Autodesk Inventor part; units mm, degrees
ref_plane "YZ Plane" through (0, 0, 0) normal (1, 0, 0) x (0, 1, 0)
ref_plane "XZ Plane" through (0, 0, 0) normal (0, 1, 0) x (-1, 0, 0)
ref_plane "XY Plane" through (0, 0, 0) normal (0, 0, 1) x (1, 0, 0)
sketch "Sketch1" plane through (0, 0, 0) normal (0, 0, 1) x (1, 0, 0)
  line L0 (0, 0) -> (25.4, 0)
  line L1 (25.4, 0) -> (25.4, 3.175)
  line L2 (3.175, 25.4) -> (0, 25.4)
  line L3 (0, 25.4) -> (0, 0)
  line L4 (3.175, 25.4) -> (3.175, 3.175)
  line L5 (3.175, 3.175) -> (25.4, 3.175)
  dimension "d1" = 25.4
  dimension "d2" = 3.175
  dimension "d3" = 3.175
  dimension "d4" = 25.4
extrude "Extrusion1" add sketch "Sketch1" along normal blind 139.7
fillet "Fillet1" radius 1.27 1 edges at (3.175, 25.4, 69.85)
fillet "Fillet2" radius 1.27 5 edges at (0, 25.4, 69.85) (25.4, 3.175, 69.85) (25.4, 0, 69.85) (0, 0, 69.85) (3.175, 3.175, 69.85)
sketch "Sketch2" plane through (4.445, 3.175, 0) normal (0, 1, 0) x (1, 0, 0)
  line L0 (0, -139.7) -> (19.685, -139.7)
  line L1 (19.685, 0) -> (0, 0)
  circle A0 centre (9.8425, -12.7) radius 3.175
  circle A1 centre (9.8425, -127) radius 3.175
  point P0 (-4.445, 0)
  dimension "d9" = 6.35
  dimension "d10" = 6.35
  dimension "d11" = 12.7
  dimension "d12" = 12.7
extrude "Extrusion2" cut sketch "Sketch2" against normal blind 152.4
sketch "Sketch3" plane through (3.175, 24.13, 139.7) normal (1, 0, 0) x (0, 0, -1)
  line L0 (44.45, -4.3683) -> (95.25, -4.3683)
  line L1 (95.25, -10.7183) -> (44.45, -10.7183)
  arc A0 (44.45, -4.3683) -> (44.45, -10.7183) centre (44.45, -7.5433) ccw
  arc A1 (95.25, -10.7183) -> (95.25, -4.3683) centre (95.25, -7.5433) ccw
  line L2 (139.7, -19.685) -> (139.7, 0)
  point P0 (139.7, -24.13)
  point P1 (0, 0)
  dimension "d20" = 44.45
  dimension "d21" = 50.8
  dimension "d22" = 139.7
extrude "Extrusion3" cut sketch "Sketch3" against normal blind 152.4
equation "\"d3\" = d2"
equation "\"d12\" = d11"
equation "\"d20\" = -0.5 * d21 + 0.5 * d22"
properties part number "BatteryMountSide"
Can you work these out from the model? Positions are in its coordinate system, mm. A direction names the side the tool comes from. Round coordinates to 2 decimals unless told otherwise and drop trailing zeros. Loops run counter-clockwise (first coordinate to the right, second up) from the corner with the lowest first, then second, coordinate; pieces in that order, holes last.
Item 1: Suppose I cut it at C-C, the plane x = 16.25. Write out the boundary of the cut face in (y, z) (3 decimals).
Item 2: Which directions (+Z, -Z, +X, -X, +Y, -Y) give clear straight access to the entire face, cutting with the end or side of a thin tool? Please do faces 4 (the flat face through (2, 13.412, 69)), 5 (the flat face through (0, 13, 69)), 6 (the flat face through (3.175, 12, 69)).
Item 3: Will these pins go through, and if not, where does the flat tip stop? pin 1 Ø8 at (x, z) = (22, 17) entering from +Y (3 decimals); pin 2 Ø5 at (x, y) = (17.5, 7) entering from -Z; pin 3 Ø12 at (y, z) = (9.5, 106.5) entering from +X; pin 4 Ø8 at (y, z) = (13.5, 19.5) entering from +X (3 decimals).
Item 4: Please list where these lines run through material, in increasing order: L1, parallel to X at y = 1.25, z = 127; L2, parallel to Z at x = 15.5, y = 2; L3, parallel to Y at x = 6, z = 30.5 (3 decimals).
Item 5: Suppose I cut it at B-B, the plane y = 17. Write out the boundary of the cut face in (x, z) (3 decimals), then the cut area to 3 significant figures.
Item 6: Suppose I cut it at D-D, the plane z = 26.5. Write out the boundary of the cut face in (x, y) (3 decimals), then the cut area to 3 significant figures.
Item 7: Suppose I cut it at A-A, the plane z = 127. Write out the boundary of the cut face in (x, y) (1 decimal).
Item 8: If we mould it in two halves opening along Z, with no side actions, what happens to faces 1 (the cylindrical face through (13.874, 1.61, 123.852)), 2 (the flat face through (14, 3.175, 69)), 3 (the flat face through (2, 7, 0))? For each: +Z half, -Z half, draft (parallel to the pull), parting line (faces both ways), or undercut.
Reported:
1. outline: (0, 0) - (3.175, 0) - (3.175, 10.204) - (0, 10.204) - close; (0, 15.196) - (3.175, 15.196) - (3.175, 124.504) - (0, 124.504) - close; (0, 129.496) - (3.175, 129.496) - (3.175, 139.7) - (0, 139.7) - close
2. face 4: +X, -X
2. face 5: +Z, -Z, -X, +Y, -Y
2. face 6: +Z, -Z, +X, +Y
3. pin 1: stops at y = 3.175
3. pin 2: passes through
3. pin 3: stops at x = 3.6
3. pin 4: stops at x = 3.175
4. L1: x = 0 to 11.11, 17.46 to 25.4
4. L2: z = 0 to 9.77, 15.63 to 124.07, 129.93 to 139.7
4. L3: y = 0 to 3.175
5. outline: (0, 0) - (3.175, 0) - (3.175, 41.302) - (0, 41.302) - close; (0, 98.398) - (3.175, 98.398) - (3.175, 139.7) - (0, 139.7) - close
5. area: 262 mm2
6. outline: (0, 1.27) arc R1.27 ccw to (1.27, 0) - (24.13, 0) arc R1.27 ccw to (25.4, 1.27) - (25.4, 1.905) arc R1.27 ccw to (24.13, 3.175) - (4.445, 3.175) arc R1.27 cw to (3.175, 4.445) - (3.175, 24.13) arc R1.27 ccw to (1.905, 25.4) - (1.27, 25.4) arc R1.27 ccw to (0, 24.13) - close
6. area: 150 mm2
7. outline: (0, 1.3) arc R1.3 ccw to (1.3, 0) - (11.1, 0) - (11.1, 3.2) - (4.4, 3.2) arc R1.3 cw to (3.2, 4.4) - (3.2, 24.1) arc R1.3 ccw to (1.9, 25.4) - (1.3, 25.4) arc R1.3 ccw to (0, 24.1) - close; (17.5, 0) - (24.1, 0) arc R1.3 ccw to (25.4, 1.3) - (25.4, 1.9) arc R1.3 ccw to (24.1, 3.2) - (17.5, 3.2) - close
8. face 1: undercut
8. face 2: draft
8. face 3: -Z half
